CAD build for the part. Positions are in the model's coordinates, mm. Face numbers are marked on the shaded views. A direction names the side the tool comes from. Coordinates: 2 decimals unless noted, no trailing zeros. Loops run counter-clockwise (first coordinate to the right, second up) from the corner with the lowest first, then second, coordinate; pieces in that order, holes last. Notation, with made-up numbers: (-3.75, 15) -> (49.25, 15) arc R25 ccw to (49.25, 33) -> close; hole circle Ø8 at (39, 0). An arc over 180 degrees is marked (long way). Return JSON: item names as keys, results as strings. Group by question number.
(1) Probe L1, parallel to Y at x = -28.5, z = 11; L2, parallel to Y at x = 16.5, z = 17.75; L3, parallel to X at y = -17.5, z = 9. List the from-to ranges inside material, lowest first.
(2) Saw through at B-B on y = 7.5. Write the cut outline in (x, z), then the cut area to 3 significant figures.
(3) Flat gauge pins, fed straight in: pin 1 Ø1.6 at (y, z) = (28, 8) entering from -X; pin 2 Ø3 at (x, y) = (-9, -23) entering from +Z; pin 3 Ø3.5 at (x, y) = (25, 26.5) entering from +Z. Where does each tip first touch, or does it go through?
(4) Saw through at A-A on x = 28. Write the cut outline in (y, z), then the cut area to 3 significant figures.
(5) Mould opens along Y. For the marked faces 1, 2, 3 and 4 say: pulls with the +Y half, pulls with the -Y half, needs draft (parallel to the pull), parting line crosses it, or undercut.
(6) Tool access for the marked faces 5 and 6: list every direction of +Z, -Z, +X, -X, +Y, -Y with a clear straight run to the whole face (end or side of a thin tool).
```python
from build123d import *

# Parameters (mm, degrees)
SKETCH_1_W            = 64
SKETCH_1_H            = 58
EXTRUDE_1_DEPTH       = 20.5
SKETCH_2_W            = 19
SKETCH_2_H            = 4.6
CUT_EXTRUDE_1_DEPTH   = 74.193237393
SKETCH_3_W            = 19
SKETCH_3_H            = 28.8
CUT_EXTRUDE_2_DEPTH   = 74.193237393
SKETCH_4_W            = 19
SKETCH_4_H            = 4.6
CUT_EXTRUDE_3_DEPTH   = 74.193237393
SKETCH_5_W            = 19
SKETCH_5_H            = 7
CUT_EXTRUDE_4_DEPTH   = 74.193237393
SKETCH_6_W            = 19
SKETCH_6_H            = 7
CUT_EXTRUDE_5_DEPTH   = 74.193237393
SKETCH_7_W            = 39.6
SKETCH_7_H            = 15.5
EXTRUDE_2_DEPTH       = 28.8
SKETCH_8_W            = 50
SKETCH_8_H            = 1.5
EXTRUDE_3_DEPTH       = 19.5
SKETCH_9_W            = 50
SKETCH_9_H            = 1.5
EXTRUDE_4_DEPTH       = 19.5
SKETCH_10_W           = 31
SKETCH_10_H           = 1.5
EXTRUDE_5_DEPTH       = 3.5
SKETCH_11_W           = 31
SKETCH_11_H           = 1.5
EXTRUDE_6_DEPTH       = 3.5
SKETCH_12_W           = 31
SKETCH_12_H           = 1.5
EXTRUDE_7_DEPTH       = 3.5
HOLE_WIZARD_6_0_6_1_D = 6
RIB_1_REACH           = 50.021
SKETCH_15_WALL_W      = 103.541657628
SKETCH_15_WALL_H      = 39.6
RIB_2_REACH           = 50.021
SKETCH_16_WALL_W      = 103.541657628
SKETCH_16_WALL_H      = 39.6
RIB_3_REACH           = 50.021
SKETCH_17_WALL_W      = 102.641657628
SKETCH_17_WALL_H      = 39.6
RIB_4_REACH           = 50.021
SKETCH_18_WALL_W      = 102.641657628
SKETCH_18_WALL_H      = 39.6
CHAMFER_1_SIZE        = 7
FILLET_1_R            = 3


with BuildPart() as part:
    # 草图1 → 凸台-拉伸1 (new body)
    with BuildSketch(Plane(origin=(0, 0, 0), x_dir=(-1, 0, 0), z_dir=(0, 0, -1))):
        Rectangle(SKETCH_1_W, SKETCH_1_H)
    extrude(amount=-EXTRUDE_1_DEPTH)

    # 草图2 → 切除-拉伸1 (cut, through all)
    with BuildSketch(Plane(origin=(32, 0, 0), x_dir=(0, 0, -1), z_dir=(1, 0, 0))):
        with Locations((-11, -18.2)):
            Rectangle(SKETCH_2_W, SKETCH_2_H)
    extrude(amount=-CUT_EXTRUDE_1_DEPTH, mode=Mode.SUBTRACT)

    # 草图3 → 切除-拉伸2 (cut, through all)
    with BuildSketch(Plane(origin=(32, 0, 0), x_dir=(0, 0, -1), z_dir=(1, 0, 0))):
        with Locations((-11, 0)):
            Rectangle(SKETCH_3_W, SKETCH_3_H)
    extrude(amount=-CUT_EXTRUDE_2_DEPTH, mode=Mode.SUBTRACT)

    # 草图4 → 切除-拉伸3 (cut, through all)
    with BuildSketch(Plane(origin=(32, 0, 0), x_dir=(0, 0, -1), z_dir=(1, 0, 0))):
        with Locations((-11, 18.2)):
            Rectangle(SKETCH_4_W, SKETCH_4_H)
    extrude(amount=-CUT_EXTRUDE_3_DEPTH, mode=Mode.SUBTRACT)

    # 草图5 → 切除-拉伸4 (cut, through all)
    with BuildSketch(Plane(origin=(32, 0, 0), x_dir=(0, 0, -1), z_dir=(1, 0, 0))):
        with Locations((-11, 25.5)):
            Rectangle(SKETCH_5_W, SKETCH_5_H)
    extrude(amount=-CUT_EXTRUDE_4_DEPTH, mode=Mode.SUBTRACT)

    # 草图6 → 切除-拉伸5 (cut, through all)
    with BuildSketch(Plane(origin=(32, 0, 0), x_dir=(0, 0, -1), z_dir=(1, 0, 0))):
        with Locations((-11, -25.5)):
            Rectangle(SKETCH_6_W, SKETCH_6_H)
    extrude(amount=-CUT_EXTRUDE_5_DEPTH, mode=Mode.SUBTRACT)

    # 草图7 → 凸台-拉伸2 (add)
    with BuildSketch(Plane.XZ.offset(-14.4)):
        with Locations((0, 9.25)):
            Rectangle(SKETCH_7_W, SKETCH_7_H)
    extrude(amount=EXTRUDE_2_DEPTH)

    # 草图8 → 凸台-拉伸3 (add)
    with BuildSketch(Plane.XY.offset(1.5)):
        with Locations((0, -28.25)):
            Rectangle(SKETCH_8_W, SKETCH_8_H)
    extrude(amount=EXTRUDE_3_DEPTH)

    # 草图9 → 凸台-拉伸4 (add)
    with BuildSketch(Plane.XY.offset(1.5)):
        with Locations((0, 28.25)):
            Rectangle(SKETCH_9_W, SKETCH_9_H)
    extrude(amount=EXTRUDE_4_DEPTH)

    # 草图10 → 凸台-拉伸5 (add)
    with BuildSketch(Plane.XY.offset(17)):
        with Locations((0.330554393, 9.05)):
            Rectangle(SKETCH_10_W, SKETCH_10_H)
    extrude(amount=EXTRUDE_5_DEPTH)

    # 草图11 → 凸台-拉伸6 (add)
    with BuildSketch(Plane.XY.offset(17)):
        with Locations((-0.104926517, -1.15574974)):
            Rectangle(SKETCH_11_W, SKETCH_11_H)
    extrude(amount=EXTRUDE_6_DEPTH)

    # 草图12 → 凸台-拉伸7 (add)
    with BuildSketch(Plane.XY.offset(17)):
        with Locations((0.330554393, -9.05)):
            Rectangle(SKETCH_12_W, SKETCH_12_H)
    extrude(amount=EXTRUDE_7_DEPTH)

    # Ø6.0 (6) 直径孔1 (through all)
    with Locations(Plane.XY.offset(1.5)):
        with Locations((28, 0), (-28, 0)):
            Hole(HOLE_WIZARD_6_0_6_1_D / 2)

    # 草图15 wall → 筋1 (add, up to next)
    with BuildSketch(Plane(origin=(0, 24.75, 17), x_dir=(0, -1, 0), z_dir=(0, 0, -1)), mode=Mode.PRIVATE) as rib_1_sk1:
        Rectangle(SKETCH_15_WALL_W, SKETCH_15_WALL_H)
    rib_1_tool1 = extrude(rib_1_sk1.sketch, amount=RIB_1_REACH, mode=Mode.PRIVATE) - part.part
    add(rib_1_tool1.solids().sort_by_distance((0, 24.75, 17))[0])

    # 草图16 wall → 筋2 (add, up to next)
    with BuildSketch(Plane(origin=(0, -24.75, 17), x_dir=(0, 1, 0), z_dir=(0, 0, -1)), mode=Mode.PRIVATE) as rib_2_sk1:
        Rectangle(SKETCH_16_WALL_W, SKETCH_16_WALL_H)
    rib_2_tool1 = extrude(rib_2_sk1.sketch, amount=RIB_2_REACH, mode=Mode.PRIVATE) - part.part
    add(rib_2_tool1.solids().sort_by_distance((0, -24.75, 17))[0])

    # 草图17 wall → 筋3 (add, up to next)
    with BuildSketch(Plane(origin=(0, 18.2, 17), x_dir=(0, 1, 0), z_dir=(0, 0, -1)), mode=Mode.PRIVATE) as rib_3_sk1:
        Rectangle(SKETCH_17_WALL_W, SKETCH_17_WALL_H)
    rib_3_tool1 = extrude(rib_3_sk1.sketch, amount=RIB_3_REACH, mode=Mode.PRIVATE) - part.part
    add(rib_3_tool1.solids().sort_by_distance((0, 18.2, 17))[0])

    # 草图18 wall → 筋4 (add, up to next)
    with BuildSketch(Plane(origin=(0, -18.2, 17), x_dir=(0, -1, 0), z_dir=(0, 0, -1)), mode=Mode.PRIVATE) as rib_4_sk1:
        Rectangle(SKETCH_18_WALL_W, SKETCH_18_WALL_H)
    rib_4_tool1 = extrude(rib_4_sk1.sketch, amount=RIB_4_REACH, mode=Mode.PRIVATE) - part.part
    add(rib_4_tool1.solids().sort_by_distance((0, -18.2, 17))[0])

    # 倒角1
    chamfer_1_edges = [part.edges().sort_by_distance(p)[0] for p in [
        (-32, 29, 0.75),
        (-32, -29, 0.75),
        (32, 29, 0.75),
        (32, -29, 0.75),
    ]]
    chamfer(chamfer_1_edges, length=CHAMFER_1_SIZE)

    # 圆角1
    fillet_1_edges = [part.edges().sort_by_distance(p)[0] for p in [
        (19.8, 0, 17),
        (-19.8, 0, 17),
        (-25, -28.25, 21),
        (25, -28.25, 21),
        (-25, 28.25, 21),
        (25, 28.25, 21),
        (-15.169445607, 9.05, 20.5),
        (15.830554393, 9.05, 20.5),
        (-32, -15.15, 20.5),
        (32, -21.25, 20.5),
        (-15.604926517, -1.15574974, 20.5),
        (15.395073483, -1.15574974, 20.5),
        (-15.169445607, -9.05, 20.5),
        (15.830554393, -9.05, 20.5),
        (19.8, 24.75, 17),
        (-19.8, 24.75, 17),
        (19.8, -24.75, 17),
        (-19.8, -24.75, 17),
        (32, -15.15, 20.5),
        (-32, 15.15, 20.5),
        (-19.8, 18.2, 17),
        (19.8, 18.2, 17),
        (-19.8, -18.2, 17),
        (19.8, -18.2, 17),
        (32, 15.15, 20.5),
        (-32, 21.25, 20.5),
        (32, 21.25, 20.5),
        (-32, -21.25, 20.5),
    ]]
    fillet(fillet_1_edges, radius=FILLET_1_R)


solid = part.part
```
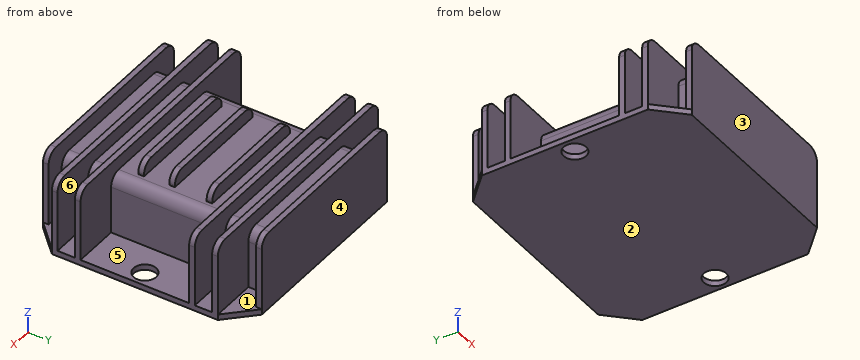
Geometry results:
{
 "1": {"L1": "-22 to -20.5, -15.9 to -14.4, 14.4 to 15.9, 20.5 to 22", "L2": "-29 to -27.5, -22 to -20.5, -15.9 to -14.4, 14.4 to 15.9, 20.5 to 22, 27.5 to 29", "L3": "-19.8 to 19.8"},
 "2": {"outline": "(-32, 0) -> (32, 0) -> (32, 1.5) -> (19.8, 1.5) -> (19.8, 14) arc R3 ccw to (16.8, 17) -> (-16.8, 17) arc R3 ccw to (-19.8, 14) -> (-19.8, 1.5) -> (-32, 1.5) -> close", "area": "706 mm²"},
 "3": {"pin 1": "x = -25", "pin 2": "z = 20.5", "pin 3": "z = 20.56"},
 "4": {"outline": "(-26, 0) -> (-3, 0) -> (-3, 1.5) -> (-14.4, 1.5) -> (-14.4, 20.5) -> (-15.9, 20.5) -> (-15.9, 1.5) -> (-20.5, 1.5) -> (-20.5, 20.5) -> (-22, 20.5) -> (-22, 1.5) -> (-26, 1.5) -> close; (3, 0) -> (26, 0) -> (26, 1.5) -> (22, 1.5) -> (22, 20.5) -> (20.5, 20.5) -> (20.5, 1.5) -> (15.9, 1.5) -> (15.9, 20.5) -> (14.4, 20.5) -> (14.4, 1.5) -> (3, 1.5) -> close", "area": "183 mm²"},
 "5": {"face 1": "undercut", "face 2": "needs draft", "face 3": "pulls with the -Y half", "face 4": "pulls with the +Y half"},
 "6": {"face 5": "+Z, +X", "face 6": "+Z"}
}
